For this review, take the finished solid that the model builds, in its own axes (mm). Face numbers are marked on the shaded views. A direction names the side the tool comes from. Coordinates: 2 decimals unless noted, no trailing zeros. Loops run counter-clockwise (first coordinate to the right, second up) from the corner with the lowest first, then second, coordinate; pieces in that order, holes last.
```python
from build123d import *

# Parameters (mm, degrees)
F1_DEPTH = 600.1512
F3_DEPTH = 0.762
F5_DEPTH = 0.762
F7_DEPTH = 0.762
F9_DEPTH = 25.4


with BuildPart() as f1:
    # F0 (on Right) → F1 (new body)
    with BuildSketch(Plane.YZ):
        Polygon((0, -151.638), (0, 0), (-0.762, 0), (-0.762, -152.4), (100.838, -152.4), (132.588, -28.620478), (131.801332, -28.620478), (100.246788, -151.638), align=None)
    extrude(amount=F1_DEPTH)

    # F2 (on face) → F3 (join)
    with BuildSketch(Plane.YZ.offset(600.1512)):
        Polygon((0, 0), (-0.762, 0), (-0.762, -152.4), (100.838, -152.4), (132.588, -28.620478), (131.801332, -28.620478), align=None)
    extrude(amount=F3_DEPTH)

    # F4 (on face) → F5 (join)
    with BuildSketch(Plane(origin=(0, 0, 0), x_dir=(0, -1, 0), z_dir=(-1, 0, 0))):
        Polygon((0.762, -152.4), (0.762, 0), (0, 0), (-131.801332, -28.620478), (-132.588, -28.620478), (-100.838, -152.4), align=None)
    extrude(amount=F5_DEPTH)

    # F6 (on face) → F7 (cut)
    with BuildSketch(Plane.XZ.offset(0.762)):
        with BuildLine():
            Line((5.588, -12.7), (5.588, -19.900739))
            ThreePointArc((5.588, -19.900739), (8.763, -31.75), (11.938, -19.900739))
            Line((11.938, -19.900739), (11.938, -12.7))
            ThreePointArc((11.938, -12.7), (8.763, -9.525), (5.588, -12.7))
        make_face()
        with BuildLine():
            ThreePointArc((588.2132, -19.900739), (591.3882, -31.75), (594.5632, -19.900739))
            Line((594.5632, -19.900739), (594.5632, -12.7))
            ThreePointArc((594.5632, -12.7), (591.3882, -9.525), (588.2132, -12.7))
            Line((588.2132, -12.7), (588.2132, -19.900739))
        make_face()
    extrude(amount=-F7_DEPTH, mode=Mode.SUBTRACT)

    # F8 (on face) → F9 (cut)
    with BuildSketch(Plane.XY.offset(-151.638)):
        with BuildLine():
            Line((84.1756, 52.621788), (58.7756, 52.621788))
            ThreePointArc((58.7756, 52.621788), (55.6006, 49.446788), (58.7756, 46.271788))
            Line((58.7756, 46.271788), (84.1756, 46.271788))
            ThreePointArc((84.1756, 46.271788), (87.3506, 49.446788), (84.1756, 52.621788))
        make_face()
        with BuildLine():
            Line((147.6756, 52.621788), (122.2756, 52.621788))
            ThreePointArc((122.2756, 52.621788), (119.1006, 49.446788), (122.2756, 46.271788))
            Line((122.2756, 46.271788), (147.6756, 46.271788))
            ThreePointArc((147.6756, 46.271788), (150.8506, 49.446788), (147.6756, 52.621788))
        make_face()
        with BuildLine():
            Line((211.1756, 52.621788), (185.7756, 52.621788))
            ThreePointArc((185.7756, 52.621788), (182.6006, 49.446788), (185.7756, 46.271788))
            Line((185.7756, 46.271788), (211.1756, 46.271788))
            ThreePointArc((211.1756, 46.271788), (214.3506, 49.446788), (211.1756, 52.621788))
        make_face()
        with BuildLine():
            Line((274.6756, 52.621788), (249.2756, 52.621788))
            ThreePointArc((249.2756, 52.621788), (246.1006, 49.446788), (249.2756, 46.271788))
            Line((249.2756, 46.271788), (274.6756, 46.271788))
            ThreePointArc((274.6756, 46.271788), (277.8506, 49.446788), (274.6756, 52.621788))
        make_face()
        with BuildLine():
            ThreePointArc((350.8756, 46.271788), (354.0506, 49.446788), (350.8756, 52.621788))
            Line((350.8756, 52.621788), (325.4756, 52.621788))
            ThreePointArc((325.4756, 52.621788), (322.3006, 49.446788), (325.4756, 46.271788))
            Line((325.4756, 46.271788), (350.8756, 46.271788))
        make_face()
        with BuildLine():
            ThreePointArc((388.9756, 52.621788), (385.8006, 49.446788), (388.9756, 46.271788))
            Line((388.9756, 46.271788), (414.3756, 46.271788))
            ThreePointArc((414.3756, 46.271788), (417.5506, 49.446788), (414.3756, 52.621788))
            Line((414.3756, 52.621788), (388.9756, 52.621788))
        make_face()
        with BuildLine():
            ThreePointArc((452.4756, 52.621788), (449.3006, 49.446788), (452.4756, 46.271788))
            Line((452.4756, 46.271788), (477.8756, 46.271788))
            ThreePointArc((477.8756, 46.271788), (481.0506, 49.446788), (477.8756, 52.621788))
            Line((477.8756, 52.621788), (452.4756, 52.621788))
        make_face()
        with BuildLine():
            ThreePointArc((541.3756, 46.271788), (544.5506, 49.446788), (541.3756, 52.621788))
            Line((541.3756, 52.621788), (515.9756, 52.621788))
            ThreePointArc((515.9756, 52.621788), (512.8006, 49.446788), (515.9756, 46.271788))
            Line((515.9756, 46.271788), (541.3756, 46.271788))
        make_face()
    extrude(amount=-F9_DEPTH, mode=Mode.SUBTRACT)


solid = f1.part
```
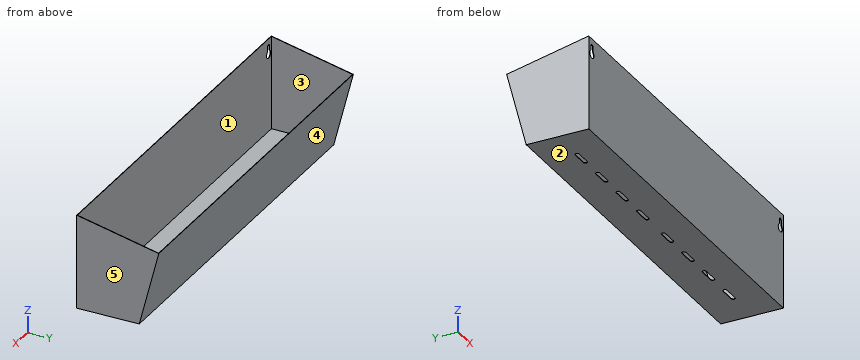
Q1. Wall thickness on probe 1 along X at (y, z) = (-0.2, -25.4); probe 2 along X at (y, z) = (93, -81.5); probe 3 along Z at (x, y) = (103.5, 89.5): over which ranges is each line inside the solid? List them lowest first.
Q2. Consider section C-C (y = 91.5). State the section outline as (x, z) points, then the cut area to 3 significant figures.
Q3. Consider section A-A (x = 523.5). State the section outline as (y, z) points.
Q4. Consider section D-D (z = -140). State the section outline as (x, y) points, then the cut area to 3 significant figures.
Q5. The part is to be moulded in two halves that separate along X. For the marked faces 3, 4 and 5, say which applies: +X half, -X half, draft (parallel to the pull), parting line (faces both ways), or undercut.
Q6. Machinability: for the marked faces 1 and 2, which of the approach directions +Z, -Z, +X, -X, +Y, -Y give a long, thin tool a straight path to every point of the face, cutting with its end or side? Answer none if there is none.
Q7. For pin 1 Ø0.6 at (x, z) = (199, -152) entering from +Y; pin 2 Ø10 at (x, y) = (483, 54) entering from +Z; pin 3 Ø20.5 at (x, z) = (8.763, -25.4) entering from -Y; pin 4 Ø12 at (x, z) = (250, -25) entering from +Y, all flat-tipped, find the tip position at first contact; note any pin that passes through.
Q8. Consider section B-B (z = -109). State the section outline as (x, y) points.
Model answer:
1. probe 1: x = -0.76 to 2.41, 15.11 to 585.04, 597.74 to 600.91
1. probe 2: x = -0.76 to 0, 600.15 to 600.91
1. probe 3: z = -152.4 to -151.64
2. outline: (-0.76, -152.4) - (600.91, -152.4) - (600.91, -19.87) - (600.15, -19.87) - (600.15, -151.64) - (0, -151.64) - (0, -19.87) - (-0.76, -19.87) - close
2. area: 659 mm2
3. outline: (-0.76, -152.4) - (46.27, -152.4) - (46.27, -151.64) - (0, -151.64) - (0, 0) - (-0.76, 0) - close; (52.62, -152.4) - (100.84, -152.4) - (132.59, -28.62) - (131.8, -28.62) - (100.25, -151.64) - (52.62, -151.64) - close
4. outline: (-0.76, -0.76) - (600.91, -0.76) - (600.91, 104.02) - (-0.76, 104.02) - close; hole (0, 0) - (600.15, 0) - (600.15, 103.23) - (0, 103.23) - close
4. area: 1,090 mm2
5. face 3: undercut
5. face 4: draft
5. face 5: +X half
6. face 1: +Z
6. face 2: -Z, +X, -X, +Y, -Y
7. pin 1: stops at y = 101.02
7. pin 2: stops at z = -151.64
7. pin 3: stops at y = -0.76
7. pin 4: stops at y = 132.59
8. outline: (-0.76, -0.76) - (600.91, -0.76) - (600.91, 111.97) - (-0.76, 111.97) - close; hole (0, 0) - (600.15, 0) - (600.15, 111.18) - (0, 111.18) - close
